Design review of the part shown in the three views and the two pictorial views. Dimensions are in mm from the part's minimum x, y and z. A direction names the side the tool comes from. Round coordinates to 2 decimals unless told otherwise and drop trailing zeros. Loops run counter-clockwise (first coordinate to the right, second up) from the corner with the lowest first, then second, coordinate; pieces in that order, holes last. Notation, with made-up numbers: M -15.75,44 L 23.25,44 A21 cw 23.25,49 Z; hole C 85,34.5 d7. An arc over 180 degrees is marked long. Return JSON: item names as keys, results as strings. Group by question number.
Q1. To check wall thickness, follow line 1 along Y through (x, z) = (94.5, 46); line 2 along X through (y, z) = (52, 54.5); line 3 along Z through (x, y) = (20, 7.5). State the ranges of each line that lie inside material, in increasing order.
Q2. Clearance check with flat-ended pins moving along their axes: pin 1 Ø1.5 at (y, z) = (22, 42.5) entering from -X; pin 2 Ø1.5 at (x, z) = (70, 57.5) entering from +Y; pin 3 Ø1.7 at (y, z) = (63, 48) entering from +X. State where each tip first meets the part, or that it passes through.
Q3. Consider section A-A (z = 63.5). State the section outline as (x, y) points, and give its area (3 significant figures).
Q4. Consider section B-B (y = 47). State the section outline as (x, z) points.
Q5. Consider section C-C (x = 87.5). State the section outline as (y, z) points.
Q6. Draft analysis for pull direction Z (two halves, no side actions). For the marked faces 3, 4 and 5, state which applies: pulls with the +Z half, pulls with the -Z half, needs draft (parallel to the pull), parting line crosses it, or undercut.
Q7. Consider section D-D (x = 8). State the section outline as (y, z) points, and give its area (3 significant figures).
Q8. For the marked faces 1 and 2, list the 3-axis set-ups (+Z, -Z, +X, -X, +Y, -Y) from which the entire face can be reached by the end or side of a thin tool; tool diameter is ignored.
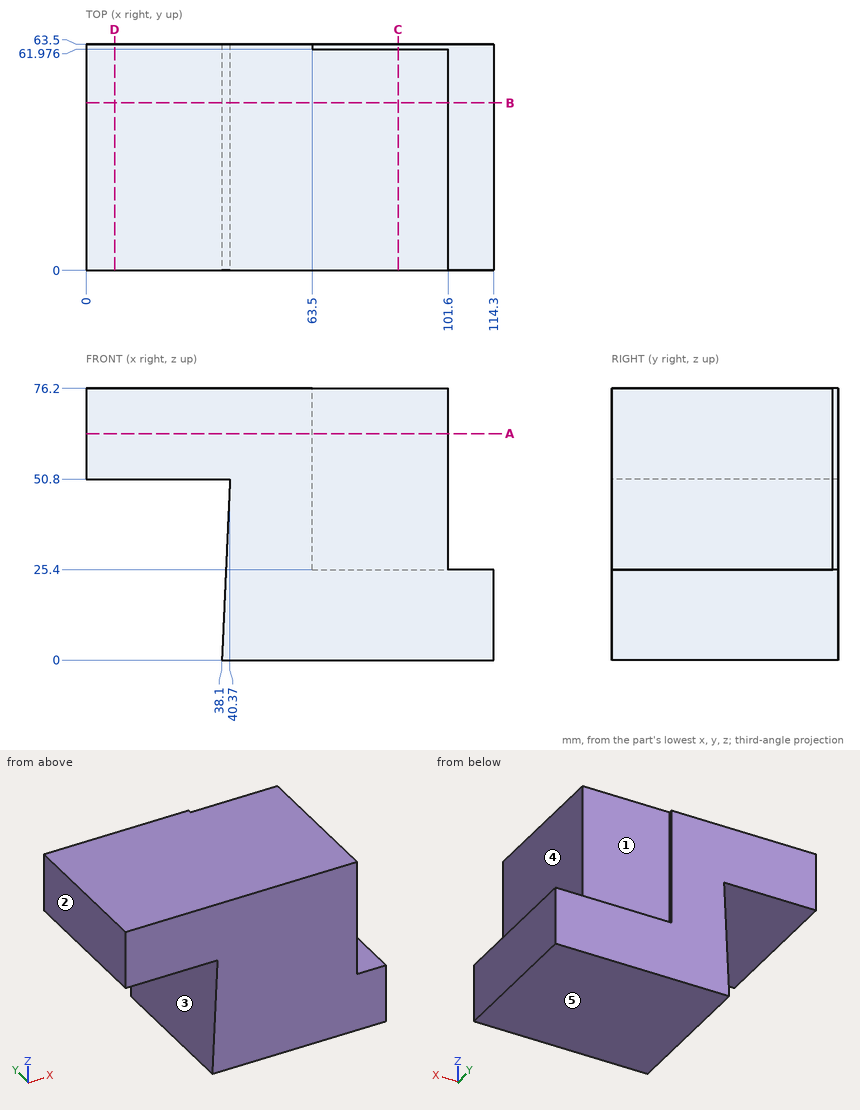
Values:
{
 "1": {"line 1": "y = 0 to 61.98", "line 2": "x = 0 to 101.6", "line 3": "z = 50.8 to 76.2"},
 "2": {"pin 1": "stops at x = 39.97", "pin 2": "stops at y = 61.98", "pin 3": "stops at x = 63.5"},
 "3": {"outline": "M 0,0 L 101.6,0 L 101.6,61.98 L 63.5,61.98 L 63.5,63.5 L 0,63.5 Z", "area": "6,390 mm2"},
 "4": {"outline": "M 0,50.8 L 40.37,50.8 L 38.1,0 L 114.3,0 L 114.3,25.4 L 101.6,25.4 L 101.6,76.2 L 0,76.2 Z"},
 "5": {"outline": "M 0,0 L 63.5,0 L 63.5,25.4 L 61.98,25.4 L 61.98,76.2 L 0,76.2 Z"},
 "6": {"face 3": "undercut", "face 4": "needs draft", "face 5": "pulls with the -Z half"},
 "7": {"outline": "M 0,50.8 L 63.5,50.8 L 63.5,76.2 L 0,76.2 Z", "area": "1,610 mm2"},
 "8": {"face 1": "+Z, +X, +Y", "face 2": "+Z, -Z, -X, +Y, -Y"}
}
